Autodesk Inventor part; units mm, degrees
ref_plane "YZ Plane" through (0, 0, 0) normal (1, 0, 0) x (0, 1, 0)
ref_plane "XZ Plane" through (0, 0, 0) normal (0, 1, 0) x (-1, 0, 0)
ref_plane "XY Plane" through (0, 0, 0) normal (0, 0, 1) x (1, 0, 0)
sketch "Esquisse7" plane through (0, 0, 0) normal (0, 0, 1) x (1, 0, 0)
  line L0 (0, -15) -> (16, -15)
  line L1 (16, -15) -> (16, 15)
  line L2 (16, 15) -> (0, 15)
  line L3 (0, 15) -> (0, -15)
  point P0 (0, 0)
  point P1 (0, 0)
  dimension "Largueur" = 16
  dimension "Hauteur" = 30
extrude "Extrusion4" add sketch "Esquisse7" along normal blind 3.8
sketch "Esquisse9" plane through (0, 15, 0) normal (0, 1, 0) x (1, 0, 0)
  arc A0 (-4, 0) -> (0, -4) centre (-4, -4) ccw
  line L0 (0, 0) -> (0, -3.8) construction
  line L1 (16, 0) -> (0, 0) construction
  line L2 (-4, 0) -> (0, 0)
  line L3 (0, 0) -> (0, -4)
  dimension "d41" = 8
extrude "Extrusion6" add sketch "Esquisse9" against normal blind 7.5
pattern_linear "Réseau rectangulaire3" count 2 spacing 15 along (0, -1, 0) of "Extrusion6"
sketch "Esquisse10" plane through (16, 15, 3.8) normal (0, 1, 0) x (1, 0, 0)
  arc A0 (-20, 3.8) -> (-16, -0.2) centre (-20, -0.2) ccw construction
  point P0 (-16, 3.8)
  point P1 (-16.0515, -0.84)
hole "Perçage2" at (-4, 15, 4) direction (0, -1, 0) diameter 3 end through all
fillet "Congé4" radius 5 2 edges at (16, 15, 1.9) (16, -15, 1.9)
sketch "Esquisse11" plane through (0, 0, 3.8) normal (0, 0, 1) x (1, 0, 0)
  line L0 (11, 15) -> (0, 15) construction
  point P0 (0, 0)
  point P1 (5.9678, 7)
  point P2 (5.9678, -7)
  point P3 (0.9356, 15)
  point P4 (5.9678, 15)
  dimension "d56" = 14
  dimension "d57" = 7
hole "Perçage3" at (5.9678, 7, 3.8) at (5.9678, -7, 3.8) direction (0, 0, -1) diameter 5 end through all countersink diameter 9 countersink angle 75
fillet "Congé5" radius 0.5 5 edges at (14.5355, 13.5355, 3.8) (16, 0, 3.8) (14.5355, -13.5355, 3.8) (5.5, -15, 3.8) (5.5, 15, 3.8)
equation "\"d42\" = 0.25 * Hauteur"
equation "\"d47\" = 0.5 * Hauteur"
equation "\"pi\" = 3.141593"
equation "\"nombredor\" = 1.61803"
properties part number "Charnière A" material "Plastique ABS"
For this review, take the finished solid that the model builds, in its own axes (mm). A direction names the side the tool comes from. Round coordinates to 2 decimals unless told otherwise and drop trailing zeros. Write each loop counter-clockwise with the first axis right and the second up, starting at its lowest first coordinate (ties: lowest second). Pieces come first, ordered by that corner, then holes. Notation, with made-up numbers: (4.25, 2) - (29.25, 2) arc R15 cw to (29.25, 27) - close; hole circle Ø3 at (-36.75, 63.25). An arc over 180 degrees is marked (long way). Use a Markdown table: item, result.
Q1. We need section C-C (z = 6). Give the boundary of the cut face in (x, y), plus the area to 3 significant figures.
Derived:
| item | result |
|---|---|
| outline | (-7.46, -7.5) - (-0.54, -7.5) - (-0.54, 0) - (-7.46, 0) - close; (-7.46, 7.5) - (-0.54, 7.5) - (-0.54, 15) - (-7.46, 15) - close |
| area | 104 mm2 |
Q2. Wall thickness on line 1 along Z through (x, y) = (-4, 13.5); line 2 along Y through (x, z) = (-2, 6); line 3 along Y through (x, z) = (5, 1): over which ranges is each line inside the solid? List them lowest first.
Derived:
| item | result |
|---|---|
| line 1 | z = 0 to 2.5, 5.5 to 8 |
| line 2 | y = -7.5 to 0, 7.5 to 15 |
| line 3 | y = -15 to -9.31, -4.69 to 4.69, 9.31 to 15 |
Q3. We need section B-B (y = 7). Give the boundary of the cut face in (x, z).
Derived:
| item | result |
|---|---|
| outline | (0, 0) - (3.47, 0) - (3.47, 1.19) - (1.47, 3.8) - (0, 3.8) - close; (8.47, 0) - (16, 0) - (16, 3.3) arc R0.5 ccw to (15.5, 3.8) - (10.47, 3.8) - (8.47, 1.19) - close |
Q4. We need section D-D (x = -3.25). Give the boundary of the cut face in (y, z).
Derived:
| item | result |
|---|---|
| outline | (-7.5, 0) - (0, 0) - (0, 2.7) - (-7.5, 2.7) - close; (-7.5, 5.3) - (0, 5.3) - (0, 7.93) - (-7.5, 7.93) - close; (7.5, 0) - (15, 0) - (15, 2.7) - (7.5, 2.7) - close; (7.5, 5.3) - (15, 5.3) - (15, 7.93) - (7.5, 7.93) - close |
Q5. We need section A-A (y = -7). Give the boundary of the cut face in (x, z).
Derived:
| item | result |
|---|---|
| outline | (-4, 0) - (3.47, 0) - (3.47, 1.19) - (1.47, 3.8) - (0, 3.8) - (0, 4) arc R4 ccw (long way) to start; (8.47, 0) - (16, 0) - (16, 3.3) arc R0.5 ccw to (15.5, 3.8) - (10.47, 3.8) - (8.47, 1.19) - close; hole circle Ø3 at (-4, 4) |
Q6. Machinability: for faces 1 (the flat face through (-2, 7.5, 4)), 2 (the flat face through (0, -11, 2)), 3 (the flat face through (8, 0, 3.8)), 4 (the flat face through (6, 0, 0)), which of the approach directions +Z, -Z, +X, -X, +Y, -Y give a long, thin tool a straight path to every point of the face, cutting with its end or side? Answer none if there is none.
Derived:
| item | result |
|---|---|
| face 1 | +Z, -Z, -X |
| face 2 | +Z, -Z, -X, -Y |
| face 3 | +Z, +X, +Y, -Y |
| face 4 | -Z, +X, -X, +Y, -Y |
Q7. Clearance check with flat-ended pins moving along their axes: pin 1 (4 mm diameter, centred on x = -4, z = 4, fed in from -Y); pin 2 (4.5 mm diameter, centred on x = 6.5, y = -4, fed in from +Z); pin 3 (1.1 mm diameter, centred on y = 4.5, z = 1, fed in from -X); pin 4 (4 mm diameter, centred on x = 5.97, y = -7, fed in from +Z) (3 decimals). State where each tip first meets the part, or that it passes through.
Derived:
| item | result |
|---|---|
| pin 1 | stops at y = -7.5 |
| pin 2 | stops at z = 3.8 |
| pin 3 | stops at x = 0 |
| pin 4 | passes through |
Q8. The part is to be moulded in two halves that separate along Y. For faces 5 (the cylindrical face through (8.186, 5.846, 0.588)), 6 (the flat face through (5, -15, 2)), 7 (the cylindrical face through (-4.45, 11.2, 5.43)), 8 (the conical face through (3.405, -6.431, 1.357)), say which applies: pulls with the +Y half, pulls with the -Y half, needs draft (parallel to the pull), parting line crosses it, or undercut.
Derived:
| item | result |
|---|---|
| face 5 | undercut |
| face 6 | pulls with the -Y half |
| face 7 | needs draft |
| face 8 | undercut |
